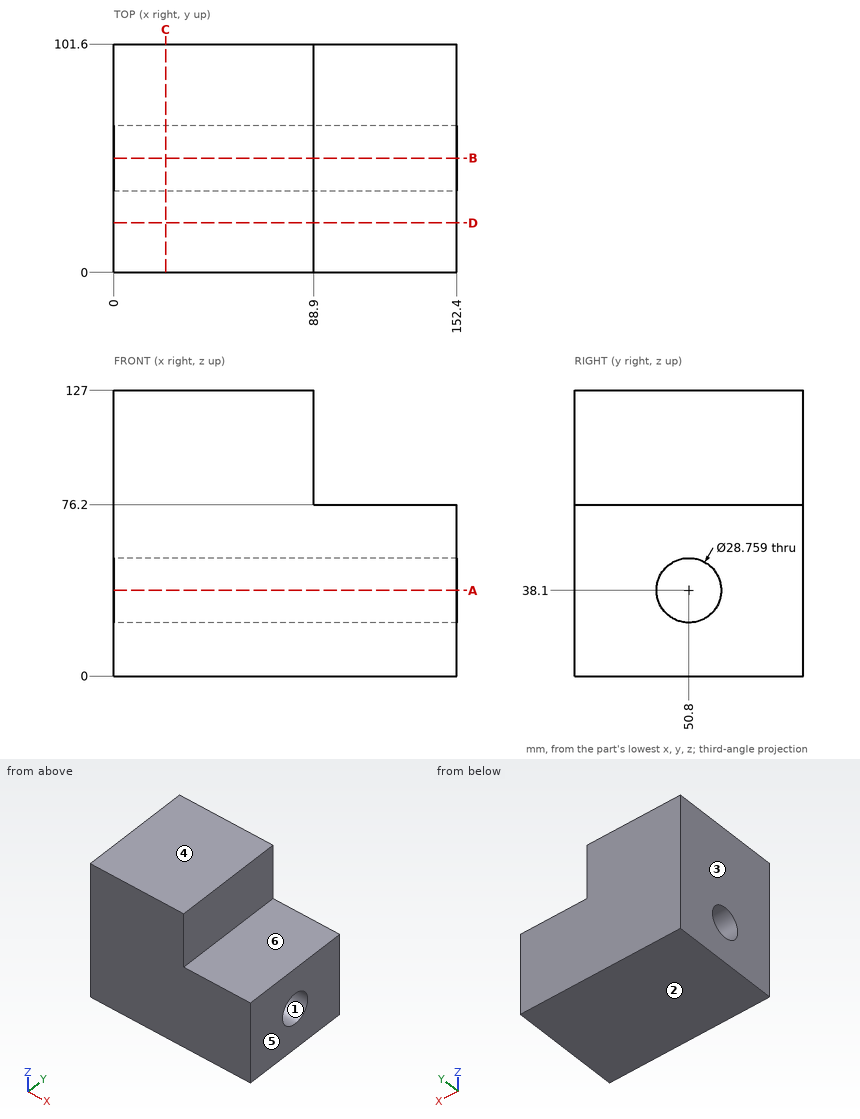
Study the drawing (mm; zero at the part's minimum x, y, z) and answer. A direction names the side the tool comes from. Round coordinates to 2 decimals unless told otherwise and drop trailing zeros. Order: outer loops, then holes, each group sorted by start corner. A loop starts at its lowest first (then second) coordinate and runs counter-clockwise, first axis right, second up. Notation, with made-up numbers: (89, -5) -> (126, -5) arc R29 cw to (126, 21) -> close; hole circle Ø1 at (5, 64.5). An arc over 180 degrees is marked (long way). Write each question's results on one line, items separated by ' | '. Start each with the question number.
Q1. Find section A-A (z = 38.1). Determine the outline of the cut face in (x, y).
Q2. Which of the six approach directions +Z, -Z, +X, -X, +Y, -Y give full straight-line access (tool end or side, diameter ignored) to the marked faces 5 and 6?
Q3. The mould has two halves that part along Z. Classify the marked faces 1, 2, 3 and 4: pulls with the +Z half, pulls with the -Z half, needs draft (parallel to the pull), parting line crosses it, or undercut.
Q4. Straight lines are drawn through the part: probe 1 along Z at (x, y) = (46, 50.8); probe 2 along Y at (x, z) = (43, 38); probe 3 along X at (y, z) = (93.5, 82). For each, find the intervals that lie inside material, in ascending order. Write a range as from..to.
Q5. Find section C-C (x = 23). Determine the outline of the cut face in (y, z).
Q6. Find section B-B (y = 50.8). Determine the outline of the cut face in (x, z).
Q7. Find section D-D (y = 22). Determine the outline of the cut face in (x, z), then the cut area to 3 significant figures.
Worked answers:
1) outline: (0, 0) -> (152.4, 0) -> (152.4, 36.42) -> (0, 36.42) -> close; (0, 65.18) -> (152.4, 65.18) -> (152.4, 101.6) -> (0, 101.6) -> close
2) face 5: +Z, -Z, +X, +Y, -Y | face 6: +Z, +X, +Y, -Y
3) face 1: undercut | face 2: pulls with the -Z half | face 3: needs draft | face 4: pulls with the +Z half
4) probe 1: z = 0..23.72, 52.48..127 | probe 2: y = 0..36.42, 65.18..101.6 | probe 3: x = 0..88.9
5) outline: (0, 0) -> (101.6, 0) -> (101.6, 127) -> (0, 127) -> close; hole circle Ø28.76 at (50.8, 38.1)
6) outline: (0, 0) -> (152.4, 0) -> (152.4, 23.72) -> (0, 23.72) -> close; (0, 52.48) -> (152.4, 52.48) -> (152.4, 76.2) -> (88.9, 76.2) -> (88.9, 127) -> (0, 127) -> close
7) outline: (0, 0) -> (152.4, 0) -> (152.4, 76.2) -> (88.9, 76.2) -> (88.9, 127) -> (0, 127) -> close | area: 16,100 mm2
